from build123d import *

# Parameters (mm, degrees)
F0_R     = 130
F0_R_2   = 1.5
F1_DEPTH = 2


with BuildPart() as f1:
    # F0 (on Front) → F1 (new body)
    with BuildSketch(Plane.XZ):
        Circle(F0_R)
        with Locations((-75.66891, -99.494804)):
            Circle(F0_R_2, mode=Mode.SUBTRACT)
        with Locations((-15.783797, -123.999483)):
            Circle(F0_R_2, mode=Mode.SUBTRACT)
        with Locations((-115.278601, -48.330573)):
            Circle(F0_R_2, mode=Mode.SUBTRACT)
        with Locations((48.330573, -115.278601)):
            Circle(F0_R_2, mode=Mode.SUBTRACT)
        with Locations((99.494804, -75.66891)):
            Circle(F0_R_2, mode=Mode.SUBTRACT)
        with Locations((123.999483, -15.783797)):
            Circle(F0_R_2, mode=Mode.SUBTRACT)
        with Locations((-123.999483, 15.783797)):
            Circle(F0_R_2, mode=Mode.SUBTRACT)
        with Locations((-99.494804, 75.66891)):
            Circle(F0_R_2, mode=Mode.SUBTRACT)
        with Locations((-48.330573, 115.278601)):
            Circle(F0_R_2, mode=Mode.SUBTRACT)
        with Locations((115.278601, 48.330573)):
            Circle(F0_R_2, mode=Mode.SUBTRACT)
        with Locations((15.783797, 123.999483)):
            Circle(F0_R_2, mode=Mode.SUBTRACT)
        with Locations((75.66891, 99.494804)):
            Circle(F0_R_2, mode=Mode.SUBTRACT)
    extrude(amount=F1_DEPTH)


solid = f1.part
Design review of the part built by this model. Coordinates are the model's own, in mm. Coordinates: 2 decimals unless noted, no trailing zeros. Order: outer loops, then holes, each group sorted by start corner. A loop starts at its lowest first (then second) coordinate and runs counter-clockwise, first axis right, second up. Notation, with made-up numbers: (-13, 88.25) -> (-9, 88.25) arc R20 ccw to (-9, 115.25) -> close; hole circle Ø7 at (27.25, -24.5). An arc over 180 degrees is marked (long way). One line per item, written item: value.
1) We need section C-C, the plane x = -82. Give the boundary of the cut face in (y, z), then the cut area to 3 significant figures.
Output values:
outline: (-2, -100.88) -> (0, -100.88) -> (0, 100.88) -> (-2, 100.88) -> close
area: 404 mm2
2) To check wall thickness, follow probe 1 along Z at (x, y) = (77, -0.25); probe 2 along X at (y, z) = (-0.3, -115.5); probe 3 along X at (y, z) = (-0.25, 57). State the ranges of each line that lie inside material, in increasing order. Write a range as [from, to].
Output values:
probe 1: z = [-104.74, 98.8], [100.19, 104.74]
probe 2: x = [-59.66, 46.85], [49.81, 59.66]
probe 3: x = [-116.84, 116.84]
3) We need section A-A, the plane y = -1.7. Count the separate pieces of the cut face and the enclosed holes in it, then the cut area to 3 significant figures.
Output values:
separate pieces: 1
enclosed holes: 12
area: 53,000 mm2
4) We need section B-B, the plane z = -55. Give the boundary of the cut face in (x, y), then the cut area to 3 significant figures.
Output values:
outline: (-117.79, -2) -> (117.79, -2) -> (117.79, 0) -> (-117.79, 0) -> close
area: 471 mm2
